from build123d import *

# Parameters (mm, degrees)
SKETCH1_W                      = 12
SKETCH1_H                      = 2
SKETCH2_R                      = 4.45
BOSS_EXTRUDE1_DEPTH            = 2.6
SKETCH3_R                      = 3.75
BOSS_EXTRUDE2_DEPTH            = 0.5
F_1_5_1_5_DIAMETER_HOLE1_D     = 1.5
F_1_5_1_5_DIAMETER_HOLE1_DEPTH = 2.5


with BuildPart() as part:
    # Sketch1 → Revolve1 (revolve)
    with BuildSketch(Plane(origin=(0, 0, 0), x_dir=(-1, 0, 0), z_dir=(0, 0, -1))):
        with Locations((-6, 1)):
            Rectangle(SKETCH1_W, SKETCH1_H)
    revolve(axis=Axis((0, 0, 0), (0, 1, 0)))

    # Sketch2 → Boss-Extrude1 (add)
    with BuildSketch(Plane.XZ):
        Circle(SKETCH2_R)
    extrude(amount=BOSS_EXTRUDE1_DEPTH)

    # Sketch3 → Boss-Extrude2 (add)
    with BuildSketch(Plane(origin=(0, 2, 0), x_dir=(-1, 0, 0), z_dir=(0, 1, 0))):
        Circle(SKETCH3_R)
    extrude(amount=BOSS_EXTRUDE2_DEPTH)

    # Sketch4 → Cut-Revolve1 (revolve, cut)
    with BuildSketch(Plane(origin=(0, 0, 0), x_dir=(-1, 0, 0), z_dir=(0, 0, -1))):
        Polygon((-2.85, -2.6), (0, -2.6), (0, 2.5), (-3, 2.5), (-3, 2), (-1.375, 2), (-1.375, 0.4), (-2.85, 0.4), align=None)
    revolve(axis=Axis((0, -2.6, 0), (0, 1, 0)), mode=Mode.SUBTRACT)

    # Ø1.5 (1.5) Diameter Hole1
    with Locations(Plane(origin=(0, 0, 0), x_dir=(-1, 0, 0), z_dir=(0, -1, 0))):
        with Locations((-9.125, 0), (9.125, 0), (-8.617750577, -3), (-8.617750577, 3), (8.617750577, -3), (8.617750577, 3), (0, 7.0625), (0, -7.0625), (-2.5, 6.605218108), (2.5, 6.605218108), (-2.5, -6.605218108), (2.5, -6.605218108), (0, 10.0625), (0, -10.0625), (-3.561946903, 9.410974472), (3.561946903, 9.410974472), (-3.561946903, -9.410974472), (3.561946903, -9.410974472)):
            Hole(F_1_5_1_5_DIAMETER_HOLE1_D / 2, depth=F_1_5_1_5_DIAMETER_HOLE1_DEPTH)


solid = part.part
Input: part model. Units: mm. Frame: model coordinates. A direction names the side the tool comes from. Coordinates: 2 decimals unless noted, no trailing zeros. Order: outer loops, then holes, each group sorted by start corner. A loop starts at its lowest first (then second) coordinate and runs counter-clockwise, first axis right, second up. Notation, with made-up numbers: M 72.5,-20.5 L 82.5,-20.5 A13 cw 82.5,-9.5 Z; hole C 64,46.25 d9. An arc over 180 degrees is marked long. One line per question, with ' | ' between items.
Item 1: Section C-C (x = -8.75). Output: boundary loops of the cut face in (y, z).
Geometry results:
outline: M 0,-8.21 L 2,-8.21 L 2,-3.74 L 0,-3.74 Z; M 0,-2.26 L 2,-2.26 L 2,-0.65 L 0,-0.65 Z; M 0,0.65 L 2,0.65 L 2,2.26 L 0,2.26 Z; M 0,3.74 L 2,3.74 L 2,8.21 L 0,8.21 Z
Item 2: Section A-A (z = 0). Give the number of separate pieces and of enclosed holes in the cut face, then the cut area to 3 significant figures.
Geometry results:
separate pieces: 4 | enclosed holes: 0 | area: 44.4 mm^2
Item 3: Ray query, line 1 along Z through (x, y) = (0, 0.9) (1 decimal); line 2 along Z through (x, y) = (3, 0.6); line 3 along Z through (x, y) = (-3.75, 0.5). Return the intervals inside material, ascending.
Geometry results:
line 1: z = -12 to -10.8, -9.3 to -7.8, -6.3 to -1.4, 1.4 to 6.3, 7.8 to 9.3, 10.8 to 12 | line 2: z = -11.62 to -9.91, -8.91 to -7.16, -6.05 to 6.05, 7.16 to 8.91, 9.91 to 11.62 | line 3: z = -11.4 to -10.14, -8.68 to 8.68, 10.14 to 11.4
Item 4: Draft query along Z for faces 3 (the flat face through (1, -2.6, -3)), 4 (the cylindrical face through (-4.115, 1.014, -9.918)), 5 (the cylindrical face through (-11.99, 1.01, -0.53)). Return one class per face: released by +Z, released by -Z, zero draft, split by the parting line, or undercut.
Geometry results:
face 3: zero draft | face 4: undercut | face 5: split by the parting line
Item 5: Pin query (flat end, axial travel): pin 1 (4 mm diameter, centred on x = -5, z = -3.5, fed in from +Y); pin 2 (2 mm diameter, centred on x = 2.5, z = -6.61, fed in from -Y); pin 3 (3 mm diameter, centred on x = 0, z = 0, fed in from -Y). Return the tip coordinate at first contact, or that it passes through.
Geometry results:
pin 1: stops at y = 2 | pin 2: stops at y = 0 | pin 3: stops at y = 0.4
Item 6: Reachability of faces 1 (the cylindrical face through (-3, 2.2, -0.1)), 2 (the cylindrical face through (-9.874, 1.014, -0.033)) from +Z, -Z, +X, -X, +Y, -Y: full face, straight path, thin tool, end or side. Return the list, or none.
Geometry results:
face 1: +Y | face 2: +Y, -Y
Item 7: Section D-D (y = -1.75). Output: boundary loops of the cut face in (x, z).
Geometry results:
outline: C 0,0 d8.9; hole C 0,0 d5.7
